Autodesk Inventor part; units mm, degrees
ref_plane "YZ Plane" through (0, 0, 0) normal (1, 0, 0) x (0, 1, 0)
ref_plane "XZ Plane" through (0, 0, 0) normal (0, 1, 0) x (-1, 0, 0)
ref_plane "XY Plane" through (0, 0, 0) normal (0, 0, 1) x (1, 0, 0)
ref_plane "作業平面1" through (-13.0598, -47.8022, -11.0593) normal (0, 1, 0) x (-1, 0, 0)
ref_plane "作業平面2" through (18.0823, -47.8022, -13) normal (0, 1, 0) x (-1, 0, 0)
sketch "スケッチ15" plane through (18.0823, -47.8022, -13) normal (0, 1, 0) x (-1, 0, 0)
  arc A0 (34.2516, 0.2523) -> (40.4568, 11) centre (24.5823, 13) ccw
  arc A1 (8.7078, 11) -> (30.7875, -1.7477) centre (24.5823, 13) ccw
  arc A2 (30.7875, 27.7477) -> (8.7078, 15) centre (24.5823, 13) ccw
  arc A3 (40.4568, 15) -> (34.2516, 25.7477) centre (24.5823, 13) ccw
  line L0 (46.5823, 11) -> (44.0823, 11)
  line L1 (44.0823, 15) -> (46.5823, 15)
  line L2 (37.0643, 30.6195) -> (36.0643, 28.8875)
  line L3 (32.6002, 30.8875) -> (33.6002, 32.6195)
  line L4 (3.0823, 15) -> (5.0823, 15)
  line L5 (5.0823, 11) -> (3.0823, 11)
  line L6 (3.0823, 11) -> (3.0823, 15)
  line L7 (46.5823, 15) -> (46.5823, 11)
  line L8 (33.6002, 32.6195) -> (37.0643, 30.6195)
  line L9 (37.3143, -5.0526) -> (33.8502, -7.0526)
  line L10 (33.8502, -7.0526) -> (32.6002, -4.8875)
  line L11 (36.0643, -2.8875) -> (37.3143, -5.0526)
  circle A4 centre (45.5823, 26) radius 1.5
  circle A5 centre (45.5823, 0) radius 1.5
  line L12 (21.5823, 36) -> (-0.4177, 19)
  line L13 (-0.4177, 19) -> (-0.4177, 7)
  line L14 (-0.4177, 7) -> (21.5823, -10)
  line L15 (49.5823, -4) -> (49.5823, 30)
  circle A6 centre (2.5823, 18) radius 1.5
  circle A7 centre (2.5823, 8) radius 1.5
  line L16 (5.0823, 11) -> (8.7078, 11)
  line L17 (5.0823, 15) -> (8.7078, 15)
  line L18 (36.0643, -2.8875) -> (34.2516, 0.2523)
  line L19 (30.7875, -1.7477) -> (32.6002, -4.8875)
  line L20 (40.4568, 11) -> (44.0823, 11)
  line L21 (44.0823, 15) -> (40.4568, 15)
  line L22 (34.2516, 25.7477) -> (36.0643, 28.8875)
  line L23 (32.6002, 30.8875) -> (30.7875, 27.7477)
  line L24 (49.5823, -4) -> (49.5823, -14)
  line L25 (49.5823, -14) -> (21.5823, -14)
  line L26 (21.5823, -14) -> (21.5823, -10)
  line L27 (21.5823, 36) -> (21.5823, 40)
  line L28 (21.5823, 40) -> (49.5823, 40)
  line L29 (49.5823, 40) -> (49.5823, 30)
  point P0 (18.0823, 13)
  dimension "d79" = 10
  dimension "d80" = 10
extrude "プレート6" add sketch "スケッチ15" along normal blind 2
chamfer "面取り4" distance 2 angle 45 4 edges at (-20.3564, -45.8022, -8) (-20.3564, -45.8022, 8) (1.5, -45.8022, 13.8564) (1.5, -45.8022, -13.8564)
sketch "スケッチ16" plane through (-31.5, -47.8022, 27) normal (0, 0, 1) x (1, 0, 0)
  point P0 (31.5, 47.8022)
sketch "スケッチ17" plane through (-31.5, -45.8022, 25) normal (0, 0, 1) x (1, 0, 0)
  line L0 (28, 0) -> (0, 0)
  line L1 (0, 0) -> (0, -8)
  line L2 (0, -8) -> (28, -8)
  line L3 (28, -8) -> (28, 0)
edge flange "フランジ2" height 8 angle 90 thickness 2 bend radius 2 thickness toward (0, 0, 1) relief straight relief width 2 relief depth 1 corner gap 2 corner form 0 edges at (-17.5, -47.8022, 27) (-17.5, -47.8022, -27) wall of the first edge with corners at (-3.5, -45.8022, 25) (-31.5, -45.8022, 25) (-31.5, -53.8022, 25) (-3.5, -53.8022, 25)
bend "曲げ2"
corner "コーナー2"
sketch "スケッチ18" plane through (-31.5, -53.8022, 27) normal (0, 0, 1) x (1, 0, 0)
  line L0 (28, 4) -> (28, 0)
  line L1 (0, 0) -> (0, 4)
  point P0 (31.5, 53.8022)
  point P1 (24, 2)
  point P2 (4, 2)
  point P3 (28, 2)
  point P4 (0, 2)
  dimension "d95" = 4
  dimension "d96" = 4
hole "穴4" at (-27.5, -51.8022, 27) at (-7.5, -51.8022, 27) direction (0, 0, -1) diameter 3 end through all
equation "\"d102\" = Thickness"
equation "\"d81\" = Thickness"
equation "\"d85\" = BendReliefWidth"
equation "\"d86\" = BendReliefDepth"
equation "\"d87\" = MinimumRemnant"
equation "\"d88\" = TransitionRadius"
equation "\"d91\" = BendRadius"
equation "\"d92\" = CornerReliefSize"
equation "\"d93\" = GapSize"
equation "\"d94\" = JacobiRadiusSize"
equation "\"BendRadius\" = Thickness"
equation "\"BendReliefWidth\" = Thickness"
equation "\"BendReliefDepth\" = 0.5 * Thickness"
equation "\"CornerReliefSize\" = 4 * Thickness"
equation "\"MinimumRemnant\" = 2 * Thickness"
equation "\"TransitionRadius\" = BendRadius"
equation "\"JacobiRadiusSize\" = Thickness"
equation "\"GapSize\" = Thickness"
properties part number "bearingcover" material "アルミニウム 6061"
Build history of the part. All positions in model axes, mm. A direction names the side the tool comes from. Coordinates: 2 decimals unless noted, no trailing zeros. Write each loop counter-clockwise with the first axis right and the second up, starting at its lowest first coordinate (ties: lowest second). Pieces come first, ordered by that corner, then holes. Notation, with made-up numbers: (68.5, -12) -> (105.5, -12) arc R27 ccw to (105.5, 27) -> close; hole circle Ø4 at (52, 48). An arc over 180 degrees is marked (long way). Use CSV: the item, a comma, the result in double quotes. Start each with the question number.
Q1. Flat gauge pins, fed straight in: pin 1 Ø2 at (y, z) = (-48.5, 26) entering from +X; pin 2 Ø2 at (x, y) = (13, -47) entering from -Z; pin 3 Ø1.5 at (x, z) = (-26, 20) entering from -Y. Where does each tip first touch, or does it go through?
Q2. 3-axis set-ups, long thin cutter, end or side, ignore diameter. For faces 4 (the flat face through (-17.52, -46.82, -19.04)), 5 (the conical face through (-20.993, -47.01, -8.48)), 6 (the flat face through (-17, -52, -25)), 7 (the cylindrical face through (-6.169, -52.494, 25.986)), 8 (the flat face through (-17, -52, -27)): which of +Z, -Z, +X, -X, +Y, -Y reach the whole face in a straight line?
Q3. Cut at A-A, the plane y = -52. List the corners of the cut face in (x, z).
Q4. Drill centre lines: probe 1 along Z at (x, y) = (-25.5, -50.5); probe 2 along Z at (x, y) = (-27.5, -46.3); probe 3 along Z at (x, y) = (-27.5, -47.4). Where is each one in solid material? Low to high.
Q5. Pull direction X, two halves, no side cores. Call faces 1 (the conical face through (1.858, -47.455, -14.049)), 2 (the flat face through (-18, -53.802, 26)), 3 (the flat face through (-3.5, -49.9, 25.5)): released by +X, released by -X, zero draft, split by the parting line, or undercut.
Q6. Cut at B-B, the plane x = -7.5. State how many separate pieces and enclosed holes the cut face has, then the cut area to 3 significant figures.
Checked values:
1,pin 1,"stops at x = -3.5"
1,pin 2,"stops at z = -11.02"
1,pin 3,"stops at y = -47.8"
2,face 4,"+Y, -Y"
2,face 5,"+Y"
2,face 6,"+X, -X, -Y"
2,face 7,"+Z, -Z"
2,face 8,"-Z, +X, -X, +Y, -Y"
3,outline,"(-31.5, -27) -> (-28.99, -27) -> (-28.99, -25) -> (-31.5, -25) -> close; (-31.5, 25) -> (-28.99, 25) -> (-28.99, 27) -> (-31.5, 27) -> close; (-26.01, -27) -> (-8.99, -27) -> (-8.99, -25) -> (-26.01, -25) -> close; (-26.01, 25) -> (-8.99, 25) -> (-8.99, 27) -> (-26.01, 27) -> close; (-6.01, -27) -> (-3.5, -27) -> (-3.5, -25) -> (-6.01, -25) -> close; (-6.01, 25) -> (-3.5, 25) -> (-3.5, 27) -> (-6.01, 27) -> close"
4,probe 1,"z = -27 to -25, 25 to 27"
4,probe 2,"z = -24.93 to -14.5, -11.5 to -2, 2 to 11.5, 14.5 to 24.93"
4,probe 3,"z = -26.2 to -14.5, -11.5 to -2, 2 to 11.5, 14.5 to 26.2"
5,face 1,"undercut"
5,face 2,"zero draft"
5,face 3,"released by +X"
6,separate pieces,"4"
6,enclosed holes,"0"
6,area,"47.0 mm²"
